```python
from build123d import *

# Parameters (mm, degrees)
SKETCH2_W           = 55
SKETCH2_H           = 12
BOSS_EXTRUDE1_DEPTH = 6
SKETCH3_W           = 25
SKETCH3_H           = 12
BOSS_EXTRUDE2_DEPTH = 13
FILLET1_R           = 5
SKETCH4_R           = 4.25
CUT_EXTRUDE2_DEPTH  = 30
SKETCH5_W           = 20.513890507
SKETCH5_H           = 7
CUT_EXTRUDE3_DEPTH  = 5
SKETCH6_R           = 1.6
CUT_EXTRUDE4_DEPTH  = 11
CUT_EXTRUDE5_DEPTH  = 3


with BuildPart() as part:
    # Sketch2 → Boss-Extrude1 (new body)
    with BuildSketch(Plane.XY):
        with Locations((27.5, 6)):
            Rectangle(SKETCH2_W, SKETCH2_H)
        with BuildLine():
            Line((6.5, 8.5), (9.5, 8.5))
            ThreePointArc((9.5, 8.5), (12, 6), (9.5, 3.5))
            Line((9.5, 3.5), (6.5, 3.5))
            ThreePointArc((6.5, 3.5), (4, 6), (6.5, 8.5))
        make_face(mode=Mode.SUBTRACT)
        with BuildLine():
            Line((48.5, 8.5), (45.5, 8.5))
            ThreePointArc((45.5, 8.5), (43, 6), (45.5, 3.5))
            Line((45.5, 3.5), (48.5, 3.5))
            ThreePointArc((48.5, 3.5), (51, 6), (48.5, 8.5))
        make_face(mode=Mode.SUBTRACT)
    extrude(amount=BOSS_EXTRUDE1_DEPTH)

    # Sketch3 → Boss-Extrude2 (add)
    with BuildSketch(Plane.XY.offset(6)):
        with Locations((27.5, 6)):
            Rectangle(SKETCH3_W, SKETCH3_H)
    extrude(amount=BOSS_EXTRUDE2_DEPTH)

    # Fillet1
    fillet1_edges = [part.edges().sort_by_distance(p)[0] for p in [
        (40, 6, 19),
    ]]
    fillet(fillet1_edges, radius=FILLET1_R)

    # Sketch4 → Cut-Extrude2 (cut)
    with BuildSketch(Plane.XZ):
        with BuildLine():
            ThreePointArc((27.86932209, 10), (27.75, 11), (27.86932209, 12))
            Line((27.86932209, 12), (15, 12))
            Line((15, 12), (15, 10))
            Line((15, 10), (27.86932209, 10))
        make_face()
        with Locations((32, 11)):
            Circle(SKETCH4_R)
    extrude(amount=-CUT_EXTRUDE2_DEPTH, mode=Mode.SUBTRACT)

    # Sketch5 → Cut-Extrude3 (cut)
    with BuildSketch(Plane(origin=(0, 0, 0), x_dir=(-1, 0, 0), z_dir=(0, 0, -1))):
        with Locations((-27.415473723, 6)):
            Rectangle(SKETCH5_W, SKETCH5_H)
    extrude(amount=-CUT_EXTRUDE3_DEPTH, mode=Mode.SUBTRACT)

    # Sketch6 → Cut-Extrude4 (cut)
    with BuildSketch(Plane.XY.offset(19)):
        with Locations((21, 6)):
            Circle(SKETCH6_R)
    extrude(amount=-CUT_EXTRUDE4_DEPTH, mode=Mode.SUBTRACT)

    # Sketch7 → Cut-Extrude5 (cut)
    with BuildSketch(Plane(origin=(0, 0, 5), x_dir=(-1, 0, 0), z_dir=(0, 0, -1))):
        Polygon((-17.535898385, 6), (-19.267949192, 9), (-22.732050808, 9), (-24.464101615, 6), (-22.732050808, 3), (-19.267949192, 3), align=None)
    extrude(amount=-CUT_EXTRUDE5_DEPTH, mode=Mode.SUBTRACT)


solid = part.part
```
Work out the finished part from the listing and answer in its coordinate system (mm). A direction names the side the tool comes from. Give positions to 0.01 mm unless a question says otherwise; leave off trailing zeros. Write each loop counter-clockwise with the first axis right and the second up, starting at its lowest first coordinate (ties: lowest second). Pieces come first, ordered by that corner, then holes. Notation, with made-up numbers: (-26, 5.5) - (2, 5.5) arc R29 cw to (2, 28.5) - close; hole circle Ø5 at (15, -27). An arc over 180 degrees is marked (long way). Use one line per item in the form item = value.
1. Each of these flat-tipped pins is pushed along its axis until it touches: pin 1 Ø7 at (x, z) = (32, 11) entering from +Y; pin 2 Ø3.5 at (y, z) = (6.5, 15) entering from -X; pin 3 Ø3.5 at (x, y) = (23.5, 7) entering from -Z; pin 4 Ø5 at (x, y) = (20.5, 6) entering from -Z. Where does it stop, or does it pass through?
Filled in:
pin_1 = through
pin_2 = 15
pin_3 = 5
pin_4 = 8
2. Consider L1, parallel to X at y = 6, z = 4.5; L2, parallel to Y at x = 26, z = 3.25; L3, parallel to Y at x = 21, z = 8.65. Determine where each line is inside the solid, lowest interval first.
Filled in:
L1 = 0 to 4, 12 to 17.16, 37.67 to 43, 51 to 55
L2 = 0 to 2.5, 9.5 to 12
L3 = 0 to 4.4, 7.6 to 12
3. A cutting plane is placed at B-B (x = 34). Write down the section's boundary in (y, z), and give its area (3 significant figures).
Filled in:
outline = (0, 0) - (2.5, 0) - (2.5, 5) - (9.5, 5) - (9.5, 0) - (12, 0) - (12, 7.25) - (0, 7.25) - close; (0, 14.75) - (12, 14.75) - (12, 19) - (0, 19) - close
area = 103 mm^2
4. A cutting plane is placed at D-D (z = 4.25). Write down the section's boundary in (x, y), and give its area (3 significant figures).
Filled in:
outline = (0, 0) - (55, 0) - (55, 12) - (0, 12) - close; hole (6.5, 3.5) - (9.5, 3.5) arc R2.5 ccw to (9.5, 8.5) - (6.5, 8.5) arc R2.5 ccw to start; hole (17.16, 2.5) - (37.67, 2.5) - (37.67, 9.5) - (17.16, 9.5) - close; hole (45.5, 3.5) - (48.5, 3.5) arc R2.5 ccw to (48.5, 8.5) - (45.5, 8.5) arc R2.5 ccw to start
area = 447 mm^2
5. A cutting plane is placed at C-C (y = 1.75). Write down the section's boundary in (x, z).
Filled in:
outline = (0, 0) - (55, 0) - (55, 6) - (40, 6) - (40, 14) arc R5 ccw to (35, 19) - (15, 19) - (15, 12) - (27.87, 12) arc R4.25 cw (long way) to (27.87, 10) - (15, 10) - (15, 6) - (0, 6) - close
6. A cutting plane is placed at A-A (z = 13). Write down the section's boundary in (x, y).
Filled in:
outline = (15, 0) - (28.25, 0) - (28.25, 12) - (15, 12) - close; (35.75, 0) - (40, 0) - (40, 12) - (35.75, 12) - close; hole circle Ø3.2 at (21, 6)
7. Determine the mould class of faces 6 (the face through (40, 6, 10)), 7 (the face through (30, 6, 5)), 8 (the face through (27, 10, 0)), 9 (the face through (37.672, 6, 2)) for opening direction X: released by +X, released by -X, zero draft, split by the parting line, or undercut.
Filled in:
face_6 = released by +X
face_7 = undercut
face_8 = zero draft
face_9 = undercut
8. For faces 1 (the face through (7, 9, 6)), 2 (the face through (4, 6, 3)), 3 (the face through (27, 0, 7)), 4 (the face through (36.246, 5.916, 10.827)), 5 (the face through (18.4, 7.5, 6.5)), determine the directions among +Z, -Z, +X, -X, +Y, -Y from which every point of the face is accessible in a straight line to the end or side of a thin tool.
Filled in:
face_1 = +Z, -X, +Y, -Y
face_2 = +Z, -Z
face_3 = +Z, -Z, +X, -X, -Y
face_4 = +Y, -Y
face_5 = -Z
